from build123d import *

# Parameters (mm, degrees)
SKETCH_1_R      = 36
SKETCH_1_R_2    = 22
SKETCH_1_R_3    = 2
EXTRUDE_1_DEPTH = 4


with BuildPart() as part:
    # 草图1 → 凸台-拉伸1 (new body)
    with BuildSketch(Plane(origin=(0, 0, 0), x_dir=(1, 0, 0), z_dir=(0, 1, 0))):
        with Locations(Location((0, 0, 0), (0, 0, 270))):
            Circle(SKETCH_1_R)
        with Locations(Location((0, 0, 0), (0, 0, 270))):
            Circle(SKETCH_1_R_2, mode=Mode.SUBTRACT)
        with Locations(Location((-25.980762114, 15, 0), (0, 0, 270))):
            Circle(SKETCH_1_R_3, mode=Mode.SUBTRACT)
        with Locations(Location((25.980762114, 15, 0), (0, 0, 270))):
            Circle(SKETCH_1_R_3, mode=Mode.SUBTRACT)
        with Locations(Location((0, -30, 0), (0, 0, 270))):
            Circle(SKETCH_1_R_3, mode=Mode.SUBTRACT)
        with BuildLine():
            ThreePointArc((-30.426663528, 8.152799921), (-31.5, 0), (-30.426663528, -8.152799921))
            ThreePointArc((-30.426663528, -8.152799921), (-27.36480135, -9.920566874), (-25.597034397, -6.858704695))
            ThreePointArc((-25.597034397, -6.858704695), (-26.5, 0), (-25.597034397, 6.858704695))
            ThreePointArc((-25.597034397, 6.858704695), (-27.36480135, 9.920566874), (-30.426663528, 8.152799921))
        make_face(mode=Mode.SUBTRACT)
        with BuildLine():
            ThreePointArc((30.426663528, 8.152799921), (31.5, 0), (30.426663528, -8.152799921))
            ThreePointArc((30.426663528, -8.152799921), (27.36480135, -9.920566874), (25.597034397, -6.858704695))
            ThreePointArc((25.597034397, -6.858704695), (26.5, 0), (25.597034397, 6.858704695))
            ThreePointArc((25.597034397, 6.858704695), (27.36480135, 9.920566874), (30.426663528, 8.152799921))
        make_face(mode=Mode.SUBTRACT)
    extrude(amount=EXTRUDE_1_DEPTH)


solid = part.part
Can you work these out from the model? Positions are in its coordinate system, mm. A direction names the side the tool comes from. Give positions to 0.01 mm unless a question says otherwise; leave off trailing zeros. Write each loop counter-clockwise with the first axis right and the second up, starting at its lowest first coordinate (ties: lowest second). Pieces come first, ordered by that corner, then holes. Notation, with made-up numbers: (36.5, -37.5) -> (88.5, -37.5) arc R23 ccw to (88.5, -8.5) -> close; hole circle Ø9 at (20, 44.25). An arc over 180 degrees is marked (long way). Answer as a JSON object with one key per item and string values. Group by question number.
Item 1: For faces 1 (the face through (-31.5, 2, -0.1)), 2 (the face through (-15, 4, -17)), which set-ups out of +Z, -Z, +X, -X, +Y, -Y let a thin tool reach every point of the face, with its end or its side?
Item 2: Please list where these lines run through material, in increasing order: line 1 (X direction, y = 2.9, z = -15); line 2 (X direction, y = 0.8, z = -8.5); line 3 (Z direction, x = -1, y = 2.2). Write a range as [from, to].
Item 3: Suppose I cut it at D-D (z = 30.5). Please give me the cut outline in (x, y).
Item 4: We'd pull the mould along X, two halves only. Please class faces 3 (the face through (-21.477, 1.972, -4.769)), 4 (the face through (10.81, 1.97, 34.34)), 5 (the face through (-15, 0, -17)), 6 (the face through (-27.418, 1.972, 9.934)): +X half, -X half, draft (parallel to the pull), parting line (faces both ways), or undercut.
Item 5: Suppose I cut it at B-B (x = 0). Please give me the cut outline in (y, z), plus the area to 3 significant figures.
Item 6: I'm going to push flat-ended pins straight in: P1, Ø3.5, axis at x = 25.98, z = -15, coming from the -Y side; P2, Ø2, axis at y = 1, z = -15.5, coming from the -X side. Where does each tip first touch, or does it pass through?
Item 7: Suppose I cut it at C-C (x = -8). Please give me the cut outline in (y, z).
Item 8: Suppose I cut it at A-A (z = 0). Please give me the cut outline in (x, y).
Findings:
{
 "1": {"face 1": "+Y, -Y", "face 2": "+Z, -Z, +X, -X, +Y"},
 "2": {"line 1": "x = [-32.73, -27.98], [-23.98, -16.09], [16.09, 23.98], [27.98, 32.73]", "line 2": "x = [-34.98, -30.31], [-25.72, -20.29], [20.29, 25.72], [30.31, 34.98]", "line 3": "z = [-35.99, -21.98], [21.98, 28.27], [31.73, 35.99]"},
 "3": {"outline": "(-19.12, 0) -> (-1.94, 0) -> (-1.94, 4) -> (-19.12, 4) -> close; (1.94, 0) -> (19.12, 0) -> (19.12, 4) -> (1.94, 4) -> close"},
 "4": {"face 3": "undercut", "face 4": "parting line", "face 5": "draft", "face 6": "undercut"},
 "5": {"outline": "(0, -36) -> (4, -36) -> (4, -22) -> (0, -22) -> close; (0, 22) -> (4, 22) -> (4, 28) -> (0, 28) -> close; (0, 32) -> (4, 32) -> (4, 36) -> (0, 36) -> close", "area": "96.0 mm²"},
 "6": {"P1": "passes through", "P2": "stops at x = -32.95"},
 "7": {"outline": "(0, -35.1) -> (4, -35.1) -> (4, -20.49) -> (0, -20.49) -> close; (0, 20.49) -> (4, 20.49) -> (4, 35.1) -> (0, 35.1) -> close"},
 "8": {"outline": "(-36, 0) -> (-31.5, 0) -> (-31.5, 4) -> (-36, 4) -> close; (-26.5, 0) -> (-22, 0) -> (-22, 4) -> (-26.5, 4) -> close; (22, 0) -> (26.5, 0) -> (26.5, 4) -> (22, 4) -> close; (31.5, 0) -> (36, 0) -> (36, 4) -> (31.5, 4) -> close"}
}
